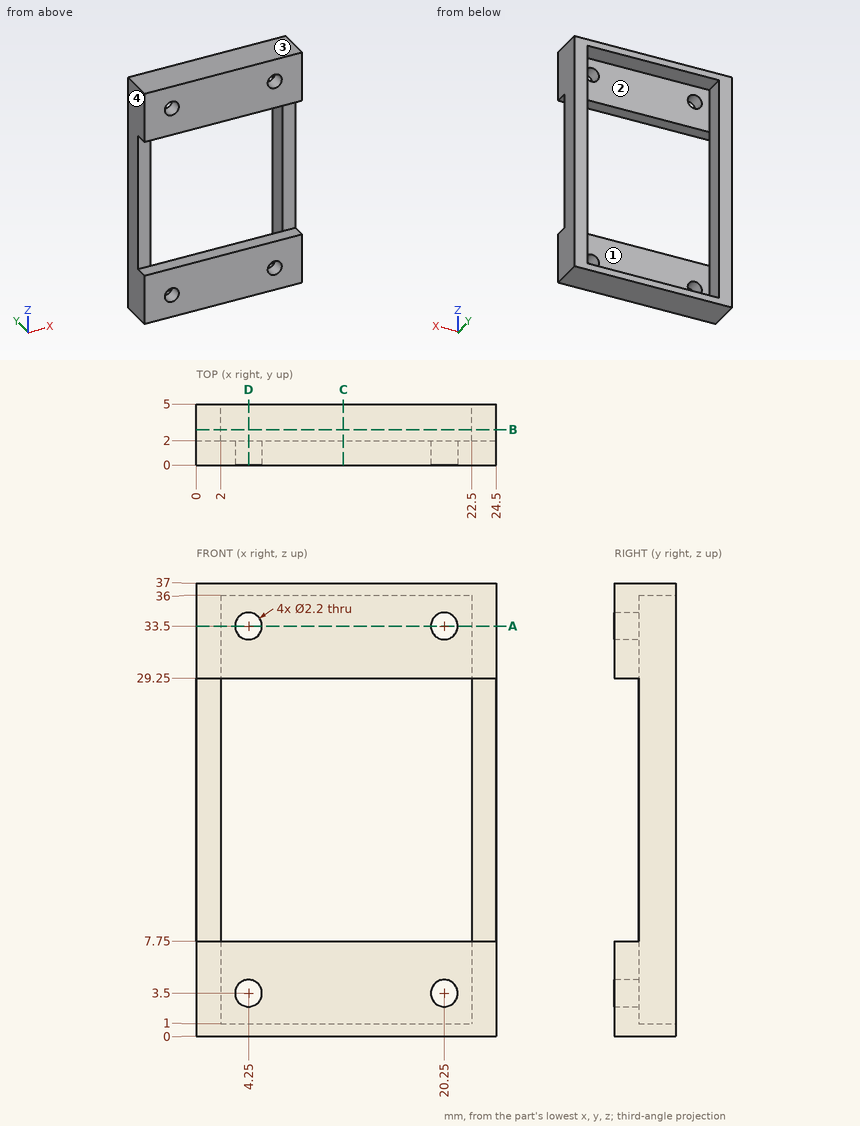
Answer from the drawing. Dimensions are ordinates in mm from the lowest x, y and z of the part. Coordinates: 2 decimals unless noted, no trailing zeros. Order: outer loops, then holes, each group sorted by start corner. A loop starts at its lowest first (then second) coordinate and runs counter-clockwise, first axis right, second up. Notation, with made-up numbers: (-25.75, 21) - (9.25, 21) arc R4 ccw to (9.25, 26) - close; hole circle Ø2 at (15.25, -36.75). An arc over 180 degrees is marked (long way). Answer as a JSON object with one key per item and string values. Group by question number.
Item 1: The mould has two halves that part along Z. Classify the marked faces 1, 2, 3 and 4: +Z half, -Z half, draft (parallel to the pull), parting line (faces both ways), or undercut.
Item 2: Flat-ended cylindrical pins translate along their axes: P1, Ø2, axis at x = 24, z = 14.5, coming from the -Y side; P2, Ø3.5, axis at x = 11, z = 31.5, coming from the +Y side. Find the tip coordinate at first contact, or state that the pin passes through.
Item 3: Section A-A (z = 33.5) is taken. Give the vertices of the cut face in (x, y).
Item 4: Section C-C (x = 12) is taken. Give the vertices of the cut face in (y, z), plus the area to 3 significant figures.
Item 5: Consider probe 1 along X at (y, z) = (0.75, 3.5); probe 2 along Z at (x, y) = (9.5, 0.5); probe 3 along X at (y, z) = (2.6, 18). Determine where each line is inside the solid, lowest interval first. Write a range as from..to.
Item 6: Section D-D (x = 4.25) is taken. Give the vertices of the cut face in (y, z), plus the area to 3 significant figures.
Item 7: Section B-B (y = 2.9) is taken. Give the vertices of the cut face in (x, z).
Results are:
{
 "1": {"face 1": "undercut", "face 2": "undercut", "face 3": "+Z half", "face 4": "draft"},
 "2": {"P1": "stops at y = 2", "P2": "stops at y = 2"},
 "3": {"outline": "(0, 0) - (3.15, 0) - (3.15, 2) - (2, 2) - (2, 5) - (0, 5) - close; (5.35, 0) - (19.15, 0) - (19.15, 2) - (5.35, 2) - close; (21.35, 0) - (24.5, 0) - (24.5, 5) - (22.5, 5) - (22.5, 2) - (21.35, 2) - close"},
 "4": {"outline": "(0, 0) - (5, 0) - (5, 1) - (2, 1) - (2, 7.75) - (0, 7.75) - close; (0, 29.25) - (2, 29.25) - (2, 36) - (5, 36) - (5, 37) - (0, 37) - close", "area": "37.0 mm^2"},
 "5": {"probe 1": "x = 0..3.15, 5.35..19.15, 21.35..24.5", "probe 2": "z = 0..7.75, 29.25..37", "probe 3": "x = 0..2, 22.5..24.5"},
 "6": {"outline": "(0, 0) - (5, 0) - (5, 1) - (2, 1) - (2, 2.4) - (0, 2.4) - close; (0, 4.6) - (2, 4.6) - (2, 7.75) - (0, 7.75) - close; (0, 29.25) - (2, 29.25) - (2, 32.4) - (0, 32.4) - close; (0, 34.6) - (2, 34.6) - (2, 36) - (5, 36) - (5, 37) - (0, 37) - close", "area": "28.2 mm^2"},
 "7": {"outline": "(0, 0) - (24.5, 0) - (24.5, 37) - (0, 37) - close; hole (2, 1) - (22.5, 1) - (22.5, 36) - (2, 36) - close"}
}
